Build history of the part. All positions in model axes, mm. A direction names the side the tool comes from. Round coordinates to 2 decimals unless told otherwise and drop trailing zeros. Write each loop counter-clockwise with the first axis right and the second up, starting at its lowest first coordinate (ties: lowest second). Pieces come first, ordered by that corner, then holes. Notation, with made-up numbers: (59, 84) -> (98, 84) arc R25 cw to (98, 113) -> close; hole circle Ø9 at (-38, 62). An arc over 180 degrees is marked (long way). Answer as CSV lines item,"result".
from build123d import *

# Parameters (mm, degrees)
SKETCH1_W           = 55
SKETCH1_H           = 54
MAINSHAPE_DEPTH     = 4.5
SKETCH2_W           = 10
SKETCH2_H           = 9
TAB1_DEPTH          = 4.5
CUT_EXTRUDE2_DEPTH  = 43.056509603
SKETCH5_W           = 4.35
SKETCH5_H           = 9.85
CUT_EXTRUDE3_DEPTH  = 43.056509603
SKETCH6_R           = 12
CUT_EXTRUDE4_DEPTH  = 43.056509603
SKETCH8_R           = 1.45
CUT_EXTRUDE6_DEPTH  = 43.056509603
SKETCH11_R          = 1.45
CUT_EXTRUDE8_DEPTH  = 43.056509603
SKETCH15_R          = 12
SKETCH15_R_2        = 6
BOSS_EXTRUDE2_DEPTH = 4.5
CUT_EXTRUDE10_DEPTH = 43.056509603
BOSS_EXTRUDE3_DEPTH = 4.5
FILLET1_R           = 3.5


with BuildPart() as part:
    # Sketch1 → MainShape (new body)
    with BuildSketch(Plane(origin=(0, 0, 0), x_dir=(1, 0, 0), z_dir=(0, 1, 0))):
        Rectangle(SKETCH1_W, SKETCH1_H)
    extrude(amount=MAINSHAPE_DEPTH)

    # Sketch2 → Tab1 (add, through all)
    with BuildSketch(Plane(origin=(0, 4.5, 0), x_dir=(1, 0, 0), z_dir=(0, 1, 0))):
        with Locations((0, 27)):
            Rectangle(SKETCH2_W, SKETCH2_H)
    extrude(amount=-TAB1_DEPTH)

    # Sketch4 → Cut-Extrude2 (cut, through all)
    with BuildSketch(Plane(origin=(0, 4.5, 0), x_dir=(1, 0, 0), z_dir=(0, 1, 0))):
        with BuildLine():
            Line((-13.45, 15), (-16.55, 15))
            Line((-16.55, 15), (-16.55, 19))
            Line((-16.55, 19), (-17.35, 19))
            ThreePointArc((-17.35, 19), (-17.703553391, 19.146446609), (-17.85, 19.5))
            Line((-17.85, 19.5), (-17.85, 22))
            ThreePointArc((-17.85, 22), (-17.703553391, 22.353553391), (-17.35, 22.5))
            Line((-17.35, 22.5), (-16.55, 22.5))
            Line((-16.55, 22.5), (-16.55, 27))
            Line((-16.55, 27), (-13.45, 27))
            Line((-13.45, 27), (-13.45, 22.5))
            Line((-13.45, 22.5), (-12.65, 22.5))
            ThreePointArc((-12.65, 22.5), (-12.296446609, 22.353553391), (-12.15, 22))
            Line((-12.15, 22), (-12.15, 19.5))
            ThreePointArc((-12.15, 19.5), (-12.296446609, 19.146446609), (-12.65, 19))
            Line((-12.65, 19), (-13.45, 19))
            Line((-13.45, 19), (-13.45, 15))
        make_face()
        with BuildLine():
            Line((13.45, 15), (13.45, 19))
            Line((13.45, 19), (12.65, 19))
            ThreePointArc((12.65, 19), (12.296446609, 19.146446609), (12.15, 19.5))
            Line((12.15, 19.5), (12.15, 22))
            ThreePointArc((12.15, 22), (12.296446609, 22.353553391), (12.65, 22.5))
            Line((12.65, 22.5), (13.45, 22.5))
            Line((13.45, 22.5), (13.45, 27))
            Line((13.45, 27), (16.55, 27))
            Line((16.55, 27), (16.55, 22.5))
            Line((16.55, 22.5), (17.35, 22.5))
            ThreePointArc((17.35, 22.5), (17.703553391, 22.353553391), (17.85, 22))
            Line((17.85, 22), (17.85, 19.5))
            ThreePointArc((17.85, 19.5), (17.703553391, 19.146446609), (17.35, 19))
            Line((17.35, 19), (16.55, 19))
            Line((16.55, 19), (16.55, 15))
            Line((16.55, 15), (13.45, 15))
        make_face()
    extrude(amount=-CUT_EXTRUDE2_DEPTH, mode=Mode.SUBTRACT)

    # Sketch5 → Cut-Extrude3 (cut, through all)
    with BuildSketch(Plane(origin=(0, 4.5, 0), x_dir=(1, 0, 0), z_dir=(0, 1, 0))):
        with Locations((23, 7)):
            Rectangle(SKETCH5_W, SKETCH5_H)
        with Locations((-23, 7)):
            Rectangle(SKETCH5_W, SKETCH5_H)
        with Locations((-23, -13)):
            Rectangle(SKETCH5_W, SKETCH5_H)
        with Locations((23, -13)):
            Rectangle(SKETCH5_W, SKETCH5_H)
    extrude(amount=-CUT_EXTRUDE3_DEPTH, mode=Mode.SUBTRACT)

    # Sketch6 → Cut-Extrude4 (cut, through all)
    with BuildSketch(Plane(origin=(0, 4.5, 0), x_dir=(1, 0, 0), z_dir=(0, 1, 0))):
        with Locations(Location((0, 1, 0), (0, 0, 270))):
            Circle(SKETCH6_R)
    extrude(amount=-CUT_EXTRUDE4_DEPTH, mode=Mode.SUBTRACT)

    # Sketch8 → Cut-Extrude6 (cut, through all)
    with BuildSketch(Plane(origin=(0, 4.5, 0), x_dir=(1, 0, 0), z_dir=(0, 1, 0))):
        with Locations(Location((-8, -20.46, 0), (0, 0, 270))):
            Circle(SKETCH8_R)
        with Locations(Location((8, -20.46, 0), (0, 0, 90))):
            Circle(SKETCH8_R)
    extrude(amount=-CUT_EXTRUDE6_DEPTH, mode=Mode.SUBTRACT)

    # Sketch11 → Cut-Extrude8 (cut, through all)
    with BuildSketch(Plane(origin=(0, 4.5, 0), x_dir=(1, 0, 0), z_dir=(0, 1, 0))):
        with Locations(Location((-23, 19.5, 0), (0, 0, 270))):
            Circle(SKETCH11_R)
        with Locations(Location((23, 19.5, 0), (0, 0, 90))):
            Circle(SKETCH11_R)
    extrude(amount=-CUT_EXTRUDE8_DEPTH, mode=Mode.SUBTRACT)

    # Sketch15 → Boss-Extrude2 (add, through all)
    with BuildSketch(Plane(origin=(0, 4.5, 0), x_dir=(1, 0, 0), z_dir=(0, 1, 0))):
        with Locations((0, 1)):
            Circle(SKETCH15_R)
        with Locations(Location((0, 1, 0), (0, 0, 270))):
            Circle(SKETCH15_R_2, mode=Mode.SUBTRACT)
    extrude(amount=-BOSS_EXTRUDE2_DEPTH)

    # Sketch16 → Cut-Extrude10 (cut, through all)
    with BuildSketch(Plane(origin=(0, 4.5, 0), x_dir=(1, 0, 0), z_dir=(0, 1, 0))):
        with BuildLine():
            Line((0, 7), (2.479202711, 7))
            ThreePointArc((2.479202711, 7), (17, 1), (2.479202711, -5))
            Line((2.479202711, -5), (0, -5))
            Line((0, -5), (0, 7))
        make_face()
    extrude(amount=-CUT_EXTRUDE10_DEPTH, mode=Mode.SUBTRACT)

    # Sketch18 → Boss-Extrude3 (add, through all)
    with BuildSketch(Plane(origin=(0, 4.5, 0), x_dir=(1, 0, 0), z_dir=(0, 1, 0))):
        with BuildLine():
            Line((-27.5, 27), (-27.55, 27))
            ThreePointArc((-27.55, 27), (-29.635965005, 27.864034995), (-30.5, 29.95))
            Line((-30.5, 29.95), (-30.5, 30))
            Line((-30.5, 30), (-33.5, 30))
            Line((-33.5, 30), (-33.5, 12))
            Line((-33.5, 12), (-30.5, 12))
            Line((-30.5, 12), (-30.5, 18.05))
            ThreePointArc((-30.5, 18.05), (-29.635965005, 20.135965005), (-27.55, 21))
            Line((-27.55, 21), (-27.5, 21))
            Line((-27.5, 21), (-27.5, 27))
        make_face()
    extrude(amount=-BOSS_EXTRUDE3_DEPTH)

    # Fillet1
    # the kernel refuses this fillet: 3.5 mm, written as the material it takes off along each edge
    with BuildSketch(Plane(origin=(-33.5, 13.160254038, -30), x_dir=(0, 0, 1), z_dir=(0, -1, 0))) as fillet1_piece_1:
        with BuildLine():
            CenterArc((3.464101615, -3.5), FILLET1_R, 90, 81.786789298)
            Line((0, -3), (-0.069282032, -2.99))
            ThreePointArc((-0.069282032, -2.99), (-0.07, -1.5), (-0.07, 0))
            Line((-0.07, 0), (0, 0.07))
            Line((0, 0.07), (3.464101615, 0.07))
            Line((3.464101615, 0.07), (3.464101615, 0))
        make_face()
    extrude(amount=21.820508076, mode=Mode.SUBTRACT)
    with BuildSketch(Plane(origin=(-33.5, 13.160254038, -12), x_dir=(1, 0, 0), z_dir=(0, -1, 0))) as fillet1_piece_2:
        with BuildLine():
            CenterArc((3.5, -3.464101615), FILLET1_R, 98.213210702, 81.786789298)
            Line((0, -3.464101615), (-0.07, -3.464101615))
            Line((-0.07, -3.464101615), (-0.07, 0))
            Line((-0.07, 0), (0, 0.07))
            ThreePointArc((0, 0.07), (1.5, 0.07), (2.99, 0.069282032))
            Line((2.99, 0.069282032), (3, 0))
        make_face()
    extrude(amount=21.820508076, mode=Mode.SUBTRACT)


solid = part.part
1. Drop flat-ended pins along their axis: pin 1 Ø2.5 at (x, z) = (8, 20.46) entering from +Y; pin 2 Ø1.6 at (x, y) = (-15.5, 2) entering from -Z; pin 3 Ø1.3 at (x, y) = (24, 3) entering from -Z; pin 4 Ø2 at (y, z) = (4, 14) entering from -X. Give the stop position or say it passes through.
Results found:
pin 1,"passes through"
pin 2,"stops at z = -15"
pin 3,"stops at z = -27"
pin 4,"stops at x = -27.5"
2. Cut at B-B, the plane x = 23. Write the cut outline in (y, z) (3 decimals).
Results found:
outline,"(0, -27) -> (4.5, -27) -> (4.5, -20.95) -> (0, -20.95) -> close; (0, -18.05) -> (4.5, -18.05) -> (4.5, -11.925) -> (0, -11.925) -> close; (0, -2.075) -> (4.5, -2.075) -> (4.5, 8.075) -> (0, 8.075) -> close; (0, 17.925) -> (4.5, 17.925) -> (4.5, 27) -> (0, 27) -> close"
3. Cut at C-C, the plane z = -10.5. Write the cut outline in (x, y) (3 decimals), then the cut area to 3 significant figures.
Results found:
outline,"(-27.5, 0) -> (-25.175, 0) -> (-25.175, 4.5) -> (-27.5, 4.5) -> close; (-20.825, 0) -> (20.825, 0) -> (20.825, 4.5) -> (-20.825, 4.5) -> close; (25.175, 0) -> (27.5, 0) -> (27.5, 4.5) -> (25.175, 4.5) -> close"
area,"208 mm2"
4. Which spindle directions (+Z, -Z, +X, -X, +Y, -Y) get a long thin tool onto all of the face, cutting with end or side? Do faces 4 (the flat face through (-16.55, 2, -25)), 5 (the flat face through (-12.15, 2, -21)), 6 (the flat face through (-27.5, 2, 3)), 7 (the flat face through (-10, 4.5, -3)). Say none if no direction does.
Results found:
face 4,"-Z, +Y, -Y"
face 5,"+Y, -Y"
face 6,"+Z, +Y, -Y"
face 7,"+Z, -Z, +X, -X, +Y"
5. Probe line 1 along X through (y, z) = (1.4, 20.46); line 2 along X through (y, z) = (2.25, -26.5); line 3 along Z through (x, y) = (8, 1.6). List the from-to ranges inside material, lowest first.
Results found:
line 1,"x = -27.5 to -9.45, -6.55 to 6.55, 9.45 to 27.5"
line 2,"x = -33.5 to -16.55, -13.45 to 13.45, 16.55 to 27.5"
line 3,"z = -27 to -9.49, 7.49 to 19.01, 21.91 to 27"
6. Mould opens along Z. For faces 1 (the flat face through (-33.5, 2, -21)), 2 (the flat face through (-22, 2, -27)), 3 (the flat face through (1, 2, 5)) say: +Z half, -Z half, draft (parallel to the pull), parting line (faces both ways), or undercut.
Results found:
face 1,"draft"
face 2,"-Z half"
face 3,"undercut"
7. Cut at D-D, the plane y = 3.75. Count the separate pieces of the cut face and the enclosed holes in it, then the cut area to 3 significant figures.
Results found:
separate pieces,"1"
enclosed holes,"9"
area,"2,500 mm2"
8. Cut at A-A, the plane x = -8. Write the cut outline in (y, z).
Results found:
outline,"(0, -27) -> (4.5, -27) -> (4.5, 19.01) -> (0, 19.01) -> close; (0, 21.91) -> (4.5, 21.91) -> (4.5, 27) -> (0, 27) -> close"
